from build123d import *

# Parameters (mm, degrees)
SKETCH1_W           = 120
SKETCH1_H           = 90
BOSS_EXTRUDE1_DEPTH = 9.5
SKETCH2_R           = 1.6
CUT_EXTRUDE1_DEPTH  = 10.5
SKETCH3_R           = 4.1
CUT_EXTRUDE2_DEPTH  = 10.5


with BuildPart() as part:
    # Sketch1 → Boss-Extrude1 (new body)
    with BuildSketch(Plane(origin=(0, 0, 0), x_dir=(1, 0, 0), z_dir=(0, 1, 0))):
        Rectangle(SKETCH1_W, SKETCH1_H)
    extrude(amount=BOSS_EXTRUDE1_DEPTH)

    # Sketch2 → Cut-Extrude1 (cut, through all)
    with BuildSketch(Plane(origin=(0, 9.5, 0), x_dir=(1, 0, 0), z_dir=(0, 1, 0))):
        with Locations((-49, -30)):
            Circle(SKETCH2_R)
        with Locations((49, -30)):
            Circle(SKETCH2_R)
        with Locations((49, 30)):
            Circle(SKETCH2_R)
        with Locations((-49, 30)):
            Circle(SKETCH2_R)
    extrude(amount=-CUT_EXTRUDE1_DEPTH, mode=Mode.SUBTRACT)

    # Sketch3 → Cut-Extrude2 (cut, through all)
    with BuildSketch(Plane(origin=(0, 9.5, 0), x_dir=(1, 0, 0), z_dir=(0, 1, 0))):
        Circle(SKETCH3_R)
    extrude(amount=-CUT_EXTRUDE2_DEPTH, mode=Mode.SUBTRACT)


solid = part.part
The model under review builds one solid part; all positions refer to its coordinate system, in mm. Round coordinates to 2 decimals unless told otherwise and drop trailing zeros. Write each loop counter-clockwise with the first axis right and the second up, starting at its lowest first coordinate (ties: lowest second). Pieces come first, ordered by that corner, then holes. Notation, with made-up numbers: (12.5, 9) - (21.5, 9) arc R25 cw to (21.5, 47) - close; hole circle Ø3 at (84.25, 87). An arc over 180 degrees is marked (long way). One line per item, written item: value. Start each with the question number.
1. Consider section C-C on z = 0. Write out the cut boundary in (x, y).
2. Consider section B-B on x = -49. Write out the cut boundary in (y, z).
3. Consider section A-A on z = -30. Write out the cut boundary in (x, y), and give its area (3 significant figures).
4. The part is to be moulded in two halves that separate along X. For faces 1 (the face through (-47.474, 4.816, -30.481)), 2 (the face through (-1, 5, 45)), 3 (the face through (60, 5, 1)), 4 (the face through (-60, 5, 1)), say which applies: released by +X, released by -X, zero draft, split by the parting line, or undercut.
5. To check wall thickness, follow L1, parallel to Z at x = -49, y = 2.5; L2, parallel to X at y = 7.5, z = -30; L3, parallel to X at y = 2, z = 0. State the ranges of each line that lie inside material, in increasing order. Write a range as from..to.
6. Clearance check with a flat-ended pin moving along its axis: P1, Ø4, axis at x = -49, z = -30, coming from the -Y side. State where the tip first meets the part, or that it passes through.
7. Consider section D-D on x = 0. Write out the cut boundary in (y, z), and give its area (3 significant figures).
Checks:
1. outline: (-60, 0) - (-4.1, 0) - (-4.1, 9.5) - (-60, 9.5) - close; (4.1, 0) - (60, 0) - (60, 9.5) - (4.1, 9.5) - close
2. outline: (0, -45) - (9.5, -45) - (9.5, -31.6) - (0, -31.6) - close; (0, -28.4) - (9.5, -28.4) - (9.5, 28.4) - (0, 28.4) - close; (0, 31.6) - (9.5, 31.6) - (9.5, 45) - (0, 45) - close
3. outline: (-60, 0) - (-50.6, 0) - (-50.6, 9.5) - (-60, 9.5) - close; (-47.4, 0) - (47.4, 0) - (47.4, 9.5) - (-47.4, 9.5) - close; (50.6, 0) - (60, 0) - (60, 9.5) - (50.6, 9.5) - close
3. area: 1,080 mm^2
4. face 1: undercut
4. face 2: zero draft
4. face 3: released by +X
4. face 4: released by -X
5. L1: z = -45..-31.6, -28.4..28.4, 31.6..45
5. L2: x = -60..-50.6, -47.4..47.4, 50.6..60
5. L3: x = -60..-4.1, 4.1..60
6. P1: stops at y = 0
7. outline: (0, -45) - (9.5, -45) - (9.5, -4.1) - (0, -4.1) - close; (0, 4.1) - (9.5, 4.1) - (9.5, 45) - (0, 45) - close
7. area: 777 mm^2
